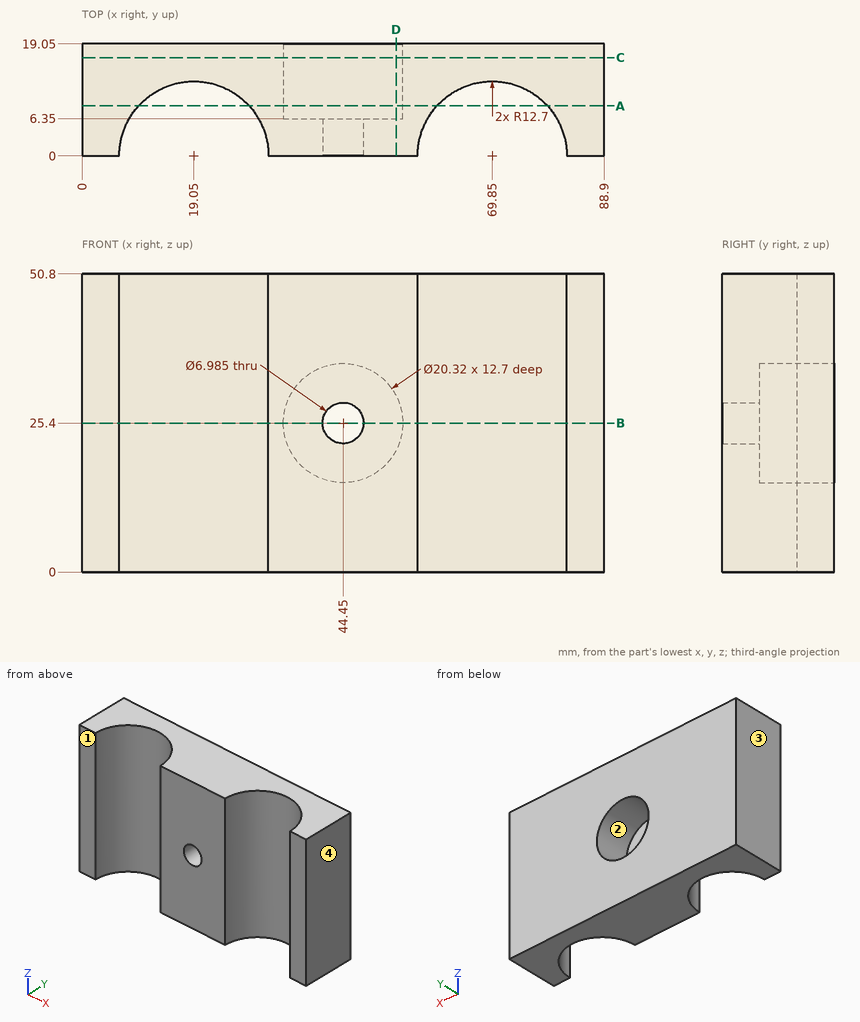
Here's the drawing with two shaded views (mm, measured from the low corner). I have some questions. Give positions to 0.01 mm unless a question says otherwise; leave off trailing zeros. Order: outer loops, then holes, each group sorted by start corner. A loop starts at its lowest first (then second) coordinate and runs counter-clockwise, first axis right, second up. Notation, with made-up numbers: (25, -32) -> (60, -32) arc R14 cw to (60, -22) -> close; hole circle Ø4 at (8.5, 44). An arc over 180 degrees is marked (long way). One line per item, written item: value. Start each with the question number.
1. We'd pull the mould along X, two halves only. Please class the marked faces 1, 2, 3 and 4: released by +X, released by -X, zero draft, split by the parting line, or undercut.
2. Imagine slicing it at B-B, the plane z = 25.4. List the corners of the cut face in (x, y) for me, plus the area to 3 significant figures.
3. Imagine slicing it at C-C, the plane y = 16.75. List the corners of the cut face in (x, z) for me.
4. I need wall thicknesses on probe 1 along X at (y, z) = (4.75, 19); probe 2 along X at (y, z) = (7.5, 13.5); probe 3 along Z at (x, y) = (44.45, 13). Which ranges of each line are inside material? Lowest first, please. Write a range as from..to.
5. Imagine slicing it at D-D, the plane x = 53.5. List the corners of the cut face in (y, z) for me.
6. Will these pins go through, and if not, where does the flat tip stop? pin 1 Ø18.5 at (x, z) = (44.45, 25.4) entering from -Y; pin 2 Ø1.5 at (x, z) = (40.5, 26) entering from +Y.
7. Imagine slicing it at A-A, the plane y = 8.5. List the corners of the cut face in (x, z) for me, plus the area to 3 significant figures.
Values follow:
1. face 1: zero draft
1. face 2: undercut
1. face 3: released by -X
1. face 4: released by +X
2. outline: (0, 0) -> (6.35, 0) arc R12.7 cw to (31.75, 0) -> (40.96, 0) -> (40.96, 6.35) -> (34.29, 6.35) -> (34.29, 19.05) -> (0, 19.05) -> close; (47.94, 0) -> (57.15, 0) arc R12.7 cw to (82.55, 0) -> (88.9, 0) -> (88.9, 19.05) -> (54.61, 19.05) -> (54.61, 6.35) -> (47.94, 6.35) -> close
2. area: 884 mm2
3. outline: (0, 0) -> (88.9, 0) -> (88.9, 50.8) -> (0, 50.8) -> close; hole circle Ø20.32 at (44.45, 25.4)
4. probe 1: x = 0..7.27, 30.83..58.07, 81.63..88.9
4. probe 2: x = 0..8.8, 29.3..59.6, 80.1..88.9
4. probe 3: z = 0..15.24, 35.56..50.8
5. outline: (0, 0) -> (19.05, 0) -> (19.05, 20.78) -> (6.35, 20.78) -> (6.35, 30.02) -> (19.05, 30.02) -> (19.05, 50.8) -> (0, 50.8) -> close
6. pin 1: stops at y = 0
6. pin 2: stops at y = 6.35
7. outline: (0, 0) -> (9.61, 0) -> (9.61, 50.8) -> (0, 50.8) -> close; (28.49, 0) -> (60.41, 0) -> (60.41, 50.8) -> (28.49, 50.8) -> close; (79.29, 0) -> (88.9, 0) -> (88.9, 50.8) -> (79.29, 50.8) -> close; hole circle Ø20.32 at (44.45, 25.4)
7. area: 2,270 mm2
